Verification items for the finished model (mm, model axes). Give positions to 0.01 mm unless a question says otherwise; leave off trailing zeros. Loops run counter-clockwise (first coordinate to the right, second up) from the corner with the lowest first, then second, coordinate; pieces in that order, holes last. Notation, with made-up numbers: M -37.75,81 L 11.25,81 A16 cw 11.25,110 Z; hole C -32,47.25 d7. An arc over 180 degrees is marked long. Use CSV: the item, a comma, the result in double quotes.
from build123d import *

# Parameters (mm, degrees)
SKETCH1_W                      = 101.6
SKETCH1_H                      = 101.6
SKETCH1_W_2                    = 95.25
SKETCH1_H_2                    = 95.25
EXTRUDE_THIN1_DEPTH            = 813
M8_CLEARANCE_HOLE2_D           = 8.4
M8_CLEARANCE_HOLE2_DEPTH       = 3.175
M8_CLEARANCE_HOLE1_D           = 9
M8_CLEARANCE_HOLE1_DEPTH       = 3.175
LPATTERN1_COUNT                = 7
LPATTERN1_PITCH                = 250
F_12_0_12_DIAMETER_HOLE1_D     = 12
F_12_0_12_DIAMETER_HOLE1_DEPTH = 3.175


with BuildPart() as part:
    # Sketch1 → Extrude-Thin1 (new, symmetric)
    with BuildSketch(Plane.XY):
        Rectangle(SKETCH1_W, SKETCH1_H)
        Rectangle(SKETCH1_W_2, SKETCH1_H_2, mode=Mode.SUBTRACT)
    extrude(amount=EXTRUDE_THIN1_DEPTH, both=True)

    # M8 Clearance Hole2
    with Locations(Plane.ZY.offset(50.8)):
        with Locations((750, 9.2), (750, -30.8)):
            m8_clearance_hole2 = Hole(M8_CLEARANCE_HOLE2_D / 2, depth=M8_CLEARANCE_HOLE2_DEPTH)

    # M8 Clearance Hole1
    with Locations(Plane.ZY.offset(-47.625)):
        with Locations((750, 9.2), (750, -30.8)):
            m8_clearance_hole1 = Hole(M8_CLEARANCE_HOLE1_D / 2, depth=M8_CLEARANCE_HOLE1_DEPTH)

    # LPattern1: M8 Clearance Hole2, M8 Clearance Hole1 ×7, 1 skipped
    with Locations(*[(0, 0, -i * LPATTERN1_PITCH) for i in range(1, LPATTERN1_COUNT) if i not in (3,)]):
        add(m8_clearance_hole2, mode=Mode.SUBTRACT)
        add(m8_clearance_hole1, mode=Mode.SUBTRACT)

    # Ø12.0 (12) Diameter Hole1
    with Locations(Plane(origin=(0, 50.8, 0), x_dir=(1, 0, 0), z_dir=(0, 1, 0))):
        with Locations((-26.2, 0), (27.8, 0)):
            Hole(F_12_0_12_DIAMETER_HOLE1_D / 2, depth=F_12_0_12_DIAMETER_HOLE1_DEPTH)


solid = part.part
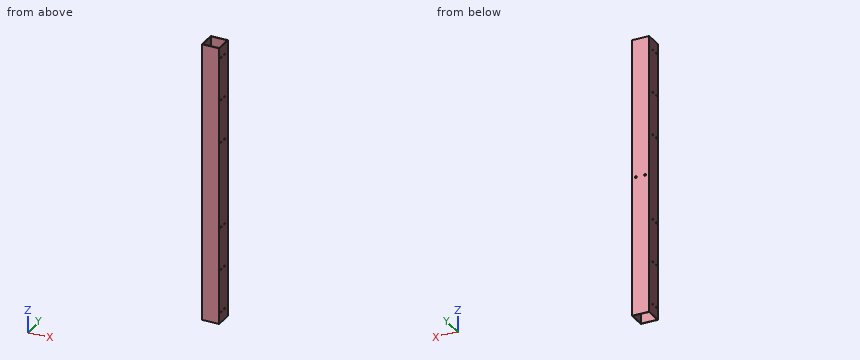
(1) Section check A-A on z = -377. Record the cut outline in (x, y) (3 decimals), plus the area to 3 significant figures.
Calculated:
outline,"M -50.8,-50.8 L 50.8,-50.8 L 50.8,50.8 L -50.8,50.8 Z; hole M -47.625,-47.625 L 47.625,-47.625 L 47.625,47.625 L -47.625,47.625 Z"
area,"1,250 mm²"
(2) Scan lines: L1, parallel to X at y = 27, z = -351.5 (3 decimals); L2, parallel to Z at x = 27.8, y = 49.1. Record each from-to range of solid material in increasing order. Write a range as from..to.
Calculated:
L1,"x = -50.8..-47.625, 47.625..50.8"
L2,"z = -813..-6, 6..813"
(3) Depth check by flat-ended pin: pin 1 Ø13.5 at (y, z) = (-30.8, -500) entering from -X; pin 2 Ø9.5 at (x, z) = (-26.2, 0) entering from +Y (3 decimals). Enter the tip coordinate at first touch or a pass-through.
Calculated:
pin 1,"stops at x = -50.8"
pin 2,"stops at y = -47.625"
